Build history of the part. All positions in model axes, mm. A direction names the side the tool comes from. Coordinates: 2 decimals unless noted, no trailing zeros. Loops run counter-clockwise (first coordinate to the right, second up) from the corner with the lowest first, then second, coordinate; pieces in that order, holes last.
(1) Flat gauge pins, fed straight in: P1, Ø9.5, axis at y = 27.5, z = -8.5, coming from the -X side; P2, Ø9.5, axis at x = 13.5, y = 15, coming from the +Z side. Where does each tip first touch, or does it go through?
(2) Slice it at A-A (z = -19.05). Give the cut face in (x, y), and give its area (3 significant figures).
(3) Wall check: L1, parallel to Y at x = 19, z = -36; L2, parallel to X at y = 24, z = -2.5; L3, parallel to Z at x = 24.5, y = 2. Give the ranges that are in metal, low to high.
(4) Slice it at D-D (x = 15). Give the cut face in (y, z).
(5) Slice it at C-C (y = 7.5). Give the cut face in (x, z).
(6) Tool access for faces 1 (the face through (38.1, 14, -19)), 2 (the face through (31.75, 18.7, -15.7)): list every direction of +Z, -Z, +X, -X, +Y, -Y with a clear straight run to the whole face (end or side of a thin tool).
(7) Two-plate mould, pull along Z, no slides. Class faces 3 (the face through (19, 14, -38.1)), 4 (the face through (34.88, 15.6, -17.58)), 5 (the face through (25, 0, -35)): pulls with the +Z half, pulls with the -Z half, needs draft (parallel to the pull), parting line crosses it, or undercut.
(8) Slice it at B-B (x = 19.05). Give the cut face in (y, z), and give its area (3 significant figures).
from build123d import *

# Parameters (mm, degrees)
SKETCH1_W           = 38.1
SKETCH1_H           = 38.1
BOSS_EXTRUDE1_DEPTH = 36.83
SKETCH2_W           = 31.75
SKETCH2_H           = 31.75
CUT_EXTRUDE1_DEPTH  = 66.266139
SKETCH4_R           = 3.175
CUT_EXTRUDE2_DEPTH  = 62.774763456
SKETCH3_R           = 3.175
CUT_EXTRUDE3_DEPTH  = 62.774763456


with BuildPart() as part:
    # Sketch1 → Boss-Extrude1 (new body)
    with BuildSketch(Plane(origin=(0, 0, 0), x_dir=(1, 0, 0), z_dir=(0, 1, 0))):
        with Locations((19.05, 19.05)):
            Rectangle(SKETCH1_W, SKETCH1_H)
    extrude(amount=BOSS_EXTRUDE1_DEPTH)

    # Sketch2 → Cut-Extrude1 (cut, through all)
    with BuildSketch(Plane(origin=(0, 36.83, 0), x_dir=(1, 0, 0), z_dir=(0, 1, 0))):
        with Locations((15.875, 15.875)):
            Rectangle(SKETCH2_W, SKETCH2_H)
    extrude(amount=-CUT_EXTRUDE1_DEPTH, mode=Mode.SUBTRACT)

    # Sketch4 → Cut-Extrude2 (cut, through all)
    with BuildSketch(Plane.ZY.offset(-31.75)):
        with Locations((-19.05, 18.415)):
            Circle(SKETCH4_R)
    extrude(amount=-CUT_EXTRUDE2_DEPTH, mode=Mode.SUBTRACT)

    # Sketch3 → Cut-Extrude3 (cut, through all)
    with BuildSketch(Plane.XY.offset(-31.75)):
        with Locations((19.05, 18.415)):
            Circle(SKETCH3_R)
    extrude(amount=-CUT_EXTRUDE3_DEPTH, mode=Mode.SUBTRACT)


solid = part.part
Response values:
1. P1: stops at x = 31.75
1. P2: stops at z = -31.75
2. outline: (31.75, 0) - (38.1, 0) - (38.1, 15.24) - (31.75, 15.24) - close; (31.75, 21.59) - (38.1, 21.59) - (38.1, 36.83) - (31.75, 36.83) - close
2. area: 194 mm2
3. L1: y = 0 to 15.24, 21.59 to 36.83
3. L2: x = 31.75 to 38.1
3. L3: z = -38.1 to -31.75
4. outline: (0, -38.1) - (36.83, -38.1) - (36.83, -31.75) - (0, -31.75) - close
5. outline: (0, -38.1) - (38.1, -38.1) - (38.1, 0) - (31.75, 0) - (31.75, -31.75) - (0, -31.75) - close
6. face 1: +Z, -Z, +X, +Y, -Y
6. face 2: +Z, -X, +Y, -Y
7. face 3: pulls with the -Z half
7. face 4: undercut
7. face 5: needs draft
8. outline: (0, -38.1) - (15.24, -38.1) - (15.24, -31.75) - (0, -31.75) - close; (21.59, -38.1) - (36.83, -38.1) - (36.83, -31.75) - (21.59, -31.75) - close
8. area: 194 mm2
